Geometry: final body of the model. Coordinates: model frame, mm. A direction names the side the tool comes from. Round coordinates to 2 decimals unless told otherwise and drop trailing zeros. Loops run counter-clockwise (first coordinate to the right, second up) from the corner with the lowest first, then second, coordinate; pieces in that order, holes last. Notation, with made-up numbers: (9, 25) - (25, 25) arc R20 ccw to (25, 61) - close; hole circle Ø6 at (-8.75, -3.5). An arc over 180 degrees is marked (long way). Write item = value, one per line. Start each with the question number.
Item 1: First-contact query: pin 1 (1 mm diameter, centred on y = -56, z = -116.5, fed in from -X); pin 2 (8 mm diameter, centred on y = -19, z = 213, fed in from +X); pin 3 (5 mm diameter, centred on y = -61, z = -52, fed in from +X). Flat tips, straight axial feed; report the tip coordinate or a pass-through.
Item 2: Draft query along X for faces 1 (the flat face through (-5, -49, -375)), 2 (the flat face through (-409.22, -49.3, -24.07)), 3 (the flat face through (419.3, -49.3, -24.2)). Return one class per face: pulls with the +X half, pulls with the -X half, needs draft (parallel to the pull), parting line crosses it, or undercut.
Item 3: Access query for faces 4 (the flat face through (-420, -100, -18)), 5 (the flat face through (5, -49, -365)). Directions: +Z, -Z, +X, -X, +Y, -Y. A direction counts if a zero-diameter tool reaches every point of the face in a straight line with its end or side. Return the directions, or none.
Item 4: Line query: line 1 (Y direction, x = -160, z = 331.5); line 2 (Z direction, x = 17.5, y = -21.5); line 3 (Y direction, x = 320, z = -370.25). Output: solid intervals per line, ascending. Write a range as from..to.
Item 5: Section C-C (z = -118). Return loops of the section in (x, y).
Item 6: Section A-A (x = -84). Return loops of the section in (y, z).
Item 7: Section B-B (y = -64). Return loops of the section in (x, z).
from build123d import *

# Parameters (mm, degrees)
F1_DEPTH = 100
F3_D     = 5
F3_DEPTH = 15
F3_TIP   = 1.5021515476
F5_D     = 10
F5_DEPTH = 15
F5_TIP   = 3.0043030951


with BuildPart() as f1:
    # F0 (on Front) → F1 (new body)
    with BuildSketch(Plane.XZ):
        Polygon((470, 336.5369722384), (-470, 336.5369722384), (-370, -375), (370, -375), align=None)
        Polygon((-458.4963159278, 326.5369722384), (458.4963159278, 326.5369722384), (361.3071326218, -365), (-361.3071326218, -365), align=None, mode=Mode.SUBTRACT)
    extrude(amount=F1_DEPTH)

    # F3
    with Locations(Plane(origin=(0, 0, -375), x_dir=(1, 0, 0), z_dir=(0, 0, -1))):
        with Locations((-320, 50), (320, 50)):
            Hole(F3_D / 2, depth=F3_DEPTH)
            with Locations((0, 0, -(F3_DEPTH + F3_TIP / 2))):  # 118° drill point
                Cone(0, F3_D / 2, F3_TIP, mode=Mode.SUBTRACT)

    # F5
    with Locations(Plane.XY.offset(336.5369722384)):
        with Locations((-410, -15), (-410, -85), (-160, -15), (-160, -85), (160, -85), (160, -15), (410, -15), (410, -85)):
            Hole(F5_D / 2, depth=F5_DEPTH)
            with Locations((0, 0, -(F5_DEPTH + F5_TIP / 2))):  # 118° drill point
                Cone(0, F5_D / 2, F5_TIP, mode=Mode.SUBTRACT)


solid = f1.part
Taken from the geometry:
q1.pin_1 = -406.4
q1.pin_2 = 453.2
q1.pin_3 = 415.75
q2.face_1 = needs draft
q2.face_2 = undercut
q2.face_3 = pulls with the +X half
q3.face_4 = +Z, -Z, +X, -X, -Y
q3.face_5 = +Y, -Y
q4.line_1 = -100..-90, -80..-20, -10..0
q4.line_2 = -375..-365, 326.54..336.54
q4.line_3 = -100..-52.5, -47.5..0
q5.outline = (-406.12, -100) - (-396.02, -100) - (-396.02, 0) - (-406.12, 0) - close; (396.02, -100) - (406.12, -100) - (406.12, 0) - (396.02, 0) - close
q6.outline = (-100, -375) - (0, -375) - (0, -365) - (-100, -365) - close; (-100, 326.54) - (0, 326.54) - (0, 336.54) - (-100, 336.54) - close
q7.outline = (-470, 336.54) - (-370, -375) - (370, -375) - (470, 336.54) - close; hole (-458.5, 326.54) - (-361.31, -365) - (361.31, -365) - (458.5, 326.54) - close
